Drawing for the job (mm, zero at the part's lowest x, y, z). A direction names the side the tool comes from. Round coordinates to 2 decimals unless told otherwise and drop trailing zeros. Loops run counter-clockwise (first coordinate to the right, second up) from the corner with the lowest first, then second, coordinate; pieces in that order, holes last. Notation, with made-up numbers: M 6,38.25 L 13,38.25 A10 ccw 13,49.25 Z; hole C 83,0 d10. An arc over 180 degrees is marked long. Use a Markdown table: item, result. Add a question column.
Q1. Pin check, flat tips, straight feed: pin 1 (11.5 mm diameter, centred on x = 21, z = 25.5, fed in from +Y); pin 2 (5 mm diameter, centred on x = 28.5, z = 30.5, fed in from -Y); pin 3 (1.5 mm diameter, centred on y = 22.5, z = 27.5, fed in from +X). Stop position of each tip, or through.
Q2. Mould opens along Z. For the marked faces 5, 6 and 7 say: +Z half, -Z half, draft (parallel to the pull), parting line (faces both ways), or undercut.
Q3. Cut at B-B (y = 29.5). Give the cut face in (x, z).
Q4. Cut at A-A (x = 17.5). State how many separate pieces and enclosed holes the cut face has.
Q5. Probe line 1 (Y direction, x = 5, z = 3); line 2 (X direction, y = 26, z = 23); line 3 (Z direction, x = 17, y = 10.5) (1 decimal). List the from-to ranges inside material, lowest first. Write a range as from..to.
Q6. Tool access for the marked faces 1, 2, 3 and 4: list every direction of +Z, -Z, +X, -X, +Y, -Y with a clear straight run to the whole face (end or side of a thin tool).
Q7. Cut at C-C (z = 31). Give the cut face in (x, y).
Q8. Cut at D-D (x = 30.5). Give the cut face in (y, z), plus the area to 3 significant figures.
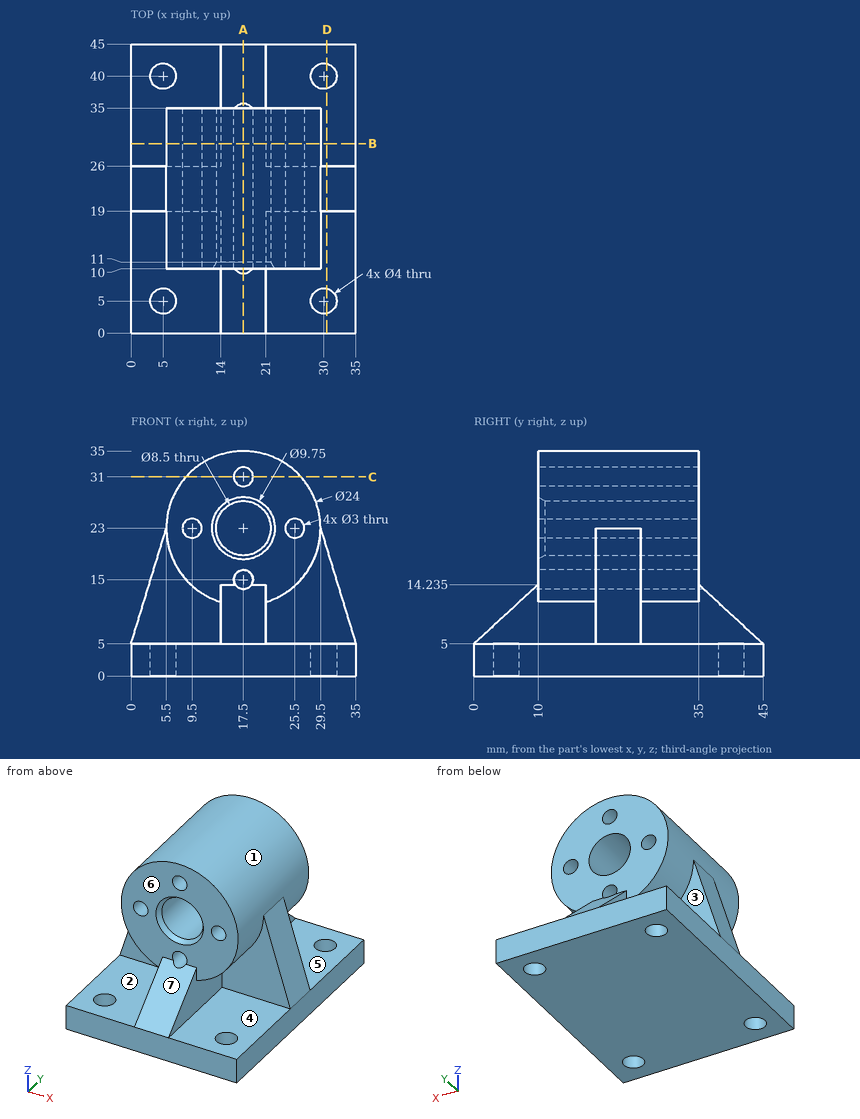
Checked values:
| question | item | result |
|---|---|---|
| 1 | pin 1 | stops at y = 35 |
| 1 | pin 2 | stops at y = 10 |
| 1 | pin 3 | stops at x = 28.9 |
| 2 | face 5 | undercut |
| 2 | face 6 | draft |
| 2 | face 7 | +Z half |
| 3 | outline | M 0,0 L 35,0 L 35,5 L 21,5 L 21,11.52 A12 ccw long 14,11.52 L 14,5 L 0,5 Z; hole C 9.5,23 d3; hole C 17.5,23 d8.5; hole C 17.5,15 d3; hole C 17.5,31 d3; hole C 25.5,23 d3 |
| 4 | separate pieces | 4 |
| 4 | enclosed holes | 0 |
| 5 | line 1 | y = 0..3, 7..38, 42..45 |
| 5 | line 2 | x = 5.5..8, 11..13.25, 21.75..24, 27..29.5 |
| 5 | line 3 | z = 0..13.6, 16.4..18.5, 27.5..29.6, 32.4..35 |
| 6 | face 1 | none |
| 6 | face 2 | -X, -Y |
| 6 | face 3 | -X, +Y |
| 6 | face 4 | +X, -Y |
| 7 | outline | M 8.56,10 L 16,10 L 16,35 L 8.56,35 Z; M 19,10 L 26.44,10 L 26.44,35 L 19,35 Z |
| 8 | outline | M 0,0 L 3.06,0 L 3.06,5 L 0,5 Z; M 6.94,0 L 38.06,0 L 38.06,5 L 26,5 L 26,19.73 L 19,19.73 L 19,5 L 6.94,5 Z; M 41.94,0 L 45,0 L 45,5 L 41.94,5 Z |
| 8 | area | 289 mm^2 |
